Autodesk Fusion 360 part; units mm, degrees
sketch "Sketch1" plane through (0, 0, 0) normal (0, 1, 0) x (1, 0, 0)
  line L0 (0, 0) -> (-82.2706, 0)
  line L1 (-82.2706, 0) -> (-82.2706, 65.5066)
  line L2 (-20.3962, 127.381) -> (0, 127.381)
  line L3 (0, 127.381) -> (0, 0)
  arc A0 (-20.3962, 127.381) -> (-82.2706, 65.5066) centre (-20.3962, 65.5066) ccw
  line L4 (-81.8896, 0.381) -> (-81.8896, 65.5066)
  arc A1 (-20.3962, 127) -> (-81.8896, 65.5066) centre (-20.3962, 65.5066) ccw
  line L5 (-20.3962, 127) -> (-0.381, 127)
  line L6 (-0.381, 127) -> (-0.381, 0.381)
  line L7 (-0.381, 0.381) -> (-81.8896, 0.381)
  dimension "d1" = 82.2706
  dimension "d2" = 127.381
  dimension "d3" = 61.8744
  dimension "d27" = -0.381
extrude "Extrude1" add sketch "Sketch1" along normal blind 76.2 contours L4 A1 L5 L6 L7 makes body 1
draft "Draft1" angle -4 neutral plane through (0, 0, 0) pull (0, 1, 0) 3 faces at (-81.8896, 25.4, -22.0895) (-81.8199, 50.8, -68.4326) (-13.7245, 25.4, -127) on bodies 1
fillet "Fillet1" radius 6.35 3 edges at (-0.381, 38.1, -129.6642) (-0.381, 38.1, -0.381) (-84.5538, 38.1, -0.381) on bodies 1
fillet "Fillet2" radius 3.175 8 edges at (-0.381, 0, -63.6827) (-2.2409, 0, -125.1356) (-13.5636, 0, -127) (-63.8786, 0, -108.989) (-81.8896, 0, -36.1188) (-80.0252, 0, -2.2409) (-41.1275, 0, -0.381) (-2.2409, 0, -2.2409) on bodies 1
shell "Shell1" thickness 1.524 removed faces 1 at (-28.4244, 76.2, -72.3421) on bodies 1
mirror "Mirror1" about plane through (0, 0, 0) normal (1, 0, 0) of bodies 1 makes body 2
delete_body "RemoveBody1" bodies 1
sketch "Sketch2" plane through (0, 76.2, 0) normal (0, 1, 0) x (-1, 0, 0)
  line L0 (-19.431, -1.905) -> (-38.481, -1.905)
  line L1 (-38.481, -1.905) -> (-38.481, -0.381)
  line L2 (-38.481, -0.381) -> (-19.431, -0.381)
  line L3 (-19.431, -0.381) -> (-19.431, -1.905)
  line L4 (-0.381, -68.8129) -> (-1.905, -68.8129)
  line L5 (-1.905, -68.8129) -> (-1.905, -113.2629)
  line L6 (-1.905, -113.2629) -> (-0.381, -113.2629)
  line L7 (-0.381, -113.2629) -> (-0.381, -68.8129)
  line L8 (-0.381, -6.731) -> (-0.381, -125.9629)
  line L9 (-1.905, -125.9629) -> (-1.905, -6.731)
  line L10 (-6.731, -1.905) -> (-80.8525, -1.905)
  line L11 (-80.8525, -0.381) -> (-6.731, -0.381)
  dimension "d17" = 19.05
  dimension "d18" = 44.45
  dimension "d32" = 12.7
  dimension "d33" = 12.7
extrude "Extrude2" cut sketch "Sketch2" against normal blind 12.7 bodies 2
draft "Draft2" angle 30 neutral plane through (0, 63.5, 0) pull (0, 1, 0) 4 faces at (38.481, 67.7333, -1.397) (1.397, 67.7333, -113.2629) (0.889, 67.7333, -68.8129) (19.431, 67.7333, -0.889) on bodies 2
fillet "Fillet3" radius 6.35 8 edges at (1.143, 76.2, -120.5953) (1.143, 63.5, -113.2629) (1.143, 76.2, -61.4806) (1.143, 63.5, -68.8129) (12.0987, 76.2, -1.143) (19.431, 63.5, -1.143) (38.481, 63.5, -1.143) (45.8133, 76.2, -1.143) on bodies 2
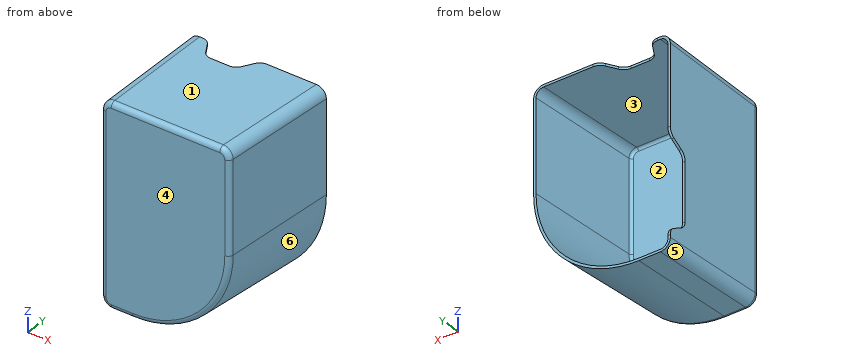
Read the model definition and answer for the solid it produces. Units are mm, in the model's axes. Face numbers are marked on the shaded views. A direction names the side the tool comes from. Round coordinates to 2 decimals unless told otherwise and drop trailing zeros. Write each loop counter-clockwise with the first axis right and the second up, starting at its lowest first coordinate (ties: lowest second). Pieces come first, ordered by that corner, then holes.
Q1. A tool of negligible diameter and unlimited length cuts with its end or side. For the marked faces 1 and 2, from which of +Z, -Z, +X, -X, +Y, -Y can it reach the whole face along a straight path? Write none if from no direction.
Values:
face 1: +Z, +X, -X, +Y, -Y
face 2: +Y
Q2. Straight lines are drawn through the part: line 1 (Y direction, x = 64, z = -89); line 2 (X direction, y = 14, z = -42) (3 decimals); line 3 (X direction, y = 73.5, z = -50) (1 decimal). For each, find the intervals that lie inside material, in ascending order.
Values:
line 1: y = 0 to 1.52
line 2: x = 0.381 to 1.905, 81.341 to 82.869
line 3: x = 0.4 to 1.9, 85.5 to 87
Q3. Find section A-A on z = -43.5. Determine the outline of the cut face in (x, y) (3 decimals), and give its area (3 significant figures).
Values:
outline: (0.381, 3.175) arc R3.175 ccw to (3.556, 0) - (78.929, 0) arc R3.175 ccw to (82.096, 2.954) - (87.218, 76.2) - (85.69, 76.2) - (80.576, 3.06) arc R1.651 cw to (78.929, 1.524) - (3.556, 1.524) arc R1.651 cw to (1.905, 3.175) - (1.905, 76.2) - (0.381, 76.2) - close
area: 349 mm2
Q4. Flat-ended cylindrical pins translate along their axes: P1, Ø2, axis at x = 68.5, y = 12.5, coming from the -Z side; P2, Ø1.2, axis at x = 30, z = -1.5, coming from the +Y side; P3, Ø1, axis at y = 62, z = -65, coming from the +X side. Find the tip coordinate at first contact, or state that the pin passes through.
Values:
P1: stops at z = -106.39
P2: stops at y = 63.5
P3: stops at x = 86.26
Q5. Find section B-B on x = 12.5. Determine the outline of the cut face in (y, z) (3 decimals).
Values:
outline: (0, -124.039) arc R3.175 ccw to (2.954, -127.207) - (76.2, -132.328) - (76.2, -130.801) - (3.06, -125.686) arc R1.651 cw to (1.524, -124.039) - (1.524, -3.556) arc R1.651 cw to (3.175, -1.905) - (74.726, -1.905) - (74.726, -0.381) - (3.175, -0.381) arc R3.175 ccw to (0, -3.556) - close
Q6. The mould has two halves that part along X. Classify the marked faces 3, 4, 5 and 6: released by +X, released by -X, zero draft, split by the parting line, or undercut.
Values:
face 3: undercut
face 4: zero draft
face 5: released by -X
face 6: released by +X
